from build123d import *

# Parameters (mm, degrees)
SKETCH1_W           = 119.38
SKETCH1_H           = 25.4
BOSS_EXTRUDE1_DEPTH = 46.355
SKETCH2_W           = 109.855
SKETCH2_H           = 83.185
CUT_EXTRUDE1_DEPTH  = 20.6375
FILLET1_R           = 2.54
FILLET2_R           = 2.54
SKETCH8_R           = 2.286
CUT_EXTRUDE2_DEPTH  = 20.32
SKETCH16_R          = 2.286
CUT_EXTRUDE4_DEPTH  = 20.32
SKETCH17_R          = 2.286
CUT_EXTRUDE5_DEPTH  = 20.32
SKETCH18_R          = 2.286
CUT_EXTRUDE6_DEPTH  = 20.32
SKETCH9_R           = 3.556
SKETCH9_R_2         = 2.286
BOSS_EXTRUDE2_DEPTH = 22.86
SKETCH11_R          = 3.556
SKETCH11_R_2        = 2.286
BOSS_EXTRUDE3_DEPTH = 22.86
SKETCH12_R          = 3.556
SKETCH12_R_2        = 2.286
BOSS_EXTRUDE4_DEPTH = 22.86
SKETCH13_R          = 3.556
SKETCH13_R_2        = 2.286
BOSS_EXTRUDE5_DEPTH = 22.86


with BuildPart() as part:
    # Sketch1 → Boss-Extrude1 (new body, symmetric)
    with BuildSketch(Plane.XY):
        with Locations((0, 12.7)):
            Rectangle(SKETCH1_W, SKETCH1_H)
    extrude(amount=BOSS_EXTRUDE1_DEPTH, both=True)

    # Sketch2 → Cut-Extrude1 (cut)
    with BuildSketch(Plane(origin=(0, 25.4, 0), x_dir=(1, 0, 0), z_dir=(0, 1, 0))):
        Rectangle(SKETCH2_W, SKETCH2_H)
    extrude(amount=-CUT_EXTRUDE1_DEPTH, mode=Mode.SUBTRACT)

    # Fillet1
    fillet1_edges = [part.edges().sort_by_distance(p)[0] for p in [
        (59.69, 12.7, 46.355),
        (-59.69, 12.7, 46.355),
        (59.69, 12.7, -46.355),
        (-59.69, 12.7, -46.355),
    ]]
    fillet(fillet1_edges, radius=FILLET1_R)

    # Fillet2
    fillet2_edges = [part.edges().sort_by_distance(p)[0] for p in [
        (59.69, 0, 0),
        (0, 0, -46.355),
        (0, 0, 46.355),
        (-59.69, 0, 0),
        (58.946051224, 0, 45.611051224),
        (-58.946051224, 0, 45.611051224),
        (-58.946051224, 0, -45.611051224),
        (58.946051224, 0, -45.611051224),
    ]]
    fillet(fillet2_edges, radius=FILLET2_R)

    # Sketch8 → Cut-Extrude2 (cut)
    with BuildSketch(Plane(origin=(0, 25.4, 0), x_dir=(1, 0, 0), z_dir=(0, 1, 0))):
        with Locations((56.896, 43.561)):
            Circle(SKETCH8_R)
    extrude(amount=-CUT_EXTRUDE2_DEPTH, mode=Mode.SUBTRACT)

    # Sketch16 → Cut-Extrude4 (cut)
    with BuildSketch(Plane(origin=(0, 25.4, 0), x_dir=(1, 0, 0), z_dir=(0, 1, 0))):
        with Locations((-56.896, -43.561)):
            Circle(SKETCH16_R)
    extrude(amount=-CUT_EXTRUDE4_DEPTH, mode=Mode.SUBTRACT)

    # Sketch17 → Cut-Extrude5 (cut)
    with BuildSketch(Plane(origin=(0, 25.4, 0), x_dir=(1, 0, 0), z_dir=(0, 1, 0))):
        with Locations((56.896, -43.561)):
            Circle(SKETCH17_R)
    extrude(amount=-CUT_EXTRUDE5_DEPTH, mode=Mode.SUBTRACT)

    # Sketch18 → Cut-Extrude6 (cut)
    with BuildSketch(Plane(origin=(0, 25.4, 0), x_dir=(1, 0, 0), z_dir=(0, 1, 0))):
        with Locations((-56.896, 43.561)):
            Circle(SKETCH18_R)
    extrude(amount=-CUT_EXTRUDE6_DEPTH, mode=Mode.SUBTRACT)

    # Sketch9 → Boss-Extrude2 (add)
    with BuildSketch(Plane(origin=(0, 4.7625, 0), x_dir=(1, 0, 0), z_dir=(0, 1, 0))):
        with Locations((-25.9715, 35.7505)):
            Circle(SKETCH9_R)
        with Locations((-25.9715, 35.7505)):
            Circle(SKETCH9_R_2, mode=Mode.SUBTRACT)
    extrude(amount=BOSS_EXTRUDE2_DEPTH)

    # Sketch11 → Boss-Extrude3 (add)
    with BuildSketch(Plane(origin=(0, 4.7625, 0), x_dir=(1, 0, 0), z_dir=(0, 1, 0))):
        with Locations((-30.8737, -32.8041)):
            Circle(SKETCH11_R)
        with Locations((-30.8737, -32.8041)):
            Circle(SKETCH11_R_2, mode=Mode.SUBTRACT)
    extrude(amount=BOSS_EXTRUDE3_DEPTH)

    # Sketch12 → Boss-Extrude4 (add)
    with BuildSketch(Plane(origin=(0, 4.7625, 0), x_dir=(1, 0, 0), z_dir=(0, 1, 0))):
        with Locations((47.8155, 35.8775)):
            Circle(SKETCH12_R)
        with Locations((47.8155, 35.8775)):
            Circle(SKETCH12_R_2, mode=Mode.SUBTRACT)
    extrude(amount=BOSS_EXTRUDE4_DEPTH)

    # Sketch13 → Boss-Extrude5 (add)
    with BuildSketch(Plane(origin=(0, 4.7625, 0), x_dir=(1, 0, 0), z_dir=(0, 1, 0))):
        with Locations((48.9585, -34.7345)):
            Circle(SKETCH13_R)
        with Locations((48.9585, -34.7345)):
            Circle(SKETCH13_R_2, mode=Mode.SUBTRACT)
    extrude(amount=BOSS_EXTRUDE5_DEPTH)


solid = part.part
Geometry check sheet. Reference: the model listing, model coordinates, mm. A direction names the side the tool comes from. Coordinates: 2 decimals unless noted, no trailing zeros. Order: outer loops, then holes, each group sorted by start corner. A loop starts at its lowest first (then second) coordinate and runs counter-clockwise, first axis right, second up. Notation, with made-up numbers: (7, -10.75) -> (19, -10.75) arc R16 ccw to (19, 19.25) -> close; hole circle Ø4 at (72.5, 68). An arc over 180 degrees is marked (long way). Use a Markdown table: item, result. Add a question column.
1. Set-up check for faces 4 (the face through (-59.69, 14, 1)), 5 (the face through (-1, 15, -41.592)): record each of +Z, -Z, +X, -X, +Y, -Y from which the full face is reachable in a straight line by a thin tool's end or side.
2. Cross-section at B-B (y = 22). Give the number of separate pieces and of enclosed holes in the cut face, and give its area (3 significant figures).
3. Material ranges on L1, parallel to Z at x = -18.5, y = 12.5 (1 decimal); L2, parallel to X at y = 11, z = -24.5; L3, parallel to Y at x = -11, z = -26.5, recorded low to high.
4. Go/stop test with flat-tipped pins: pin 1 Ø2.5 at (x, z) = (57, 43) entering from +Y; pin 2 Ø2.5 at (x, z) = (48.5, -35.5) entering from +Y; pin 3 Ø5.5 at (x, z) = (56.896, -43.561) entering from +Y. Record where each tip stops, or that it passes through.
5. Cross-section at A-A (z = 0). Enter the section's corners in (x, y).
6. Mould release check, pull along Z, two halves, no side actions. Record for faces 1 (the face through (59.69, 14, 1)), 2 (the face through (-57, 5.08, -44)), 3 (the face through (0.8, 0.724, -45.591)): pulls with the +Z half, pulls with the -Z half, needs draft (parallel to the pull), parting line crosses it, or undercut.
7. Cross-section at C-C (x = 16). Enter the section's corners in (y, z) (1 decimal).
Filled sheet:
| question | item | result |
|---|---|---|
| 1 | face 4 | +Z, -Z, -X, +Y, -Y |
| 1 | face 5 | +Y |
| 2 | separate pieces | 5 |
| 2 | enclosed holes | 9 |
| 2 | area | 1,950 mm2 |
| 3 | L1 | -46.4 to -41.6, 41.6 to 46.4 |
| 3 | L2 | -59.69 to -54.93, 54.93 to 59.69 |
| 3 | L3 | 0 to 4.76 |
| 4 | pin 1 | y = 5.08 |
| 4 | pin 2 | y = 4.76 |
| 4 | pin 3 | y = 25.4 |
| 5 | outline | (-59.69, 2.54) arc R2.54 ccw to (-57.15, 0) -> (57.15, 0) arc R2.54 ccw to (59.69, 2.54) -> (59.69, 25.4) -> (54.93, 25.4) -> (54.93, 4.76) -> (-54.93, 4.76) -> (-54.93, 25.4) -> (-59.69, 25.4) -> close |
| 6 | face 1 | needs draft |
| 6 | face 2 | undercut |
| 6 | face 3 | pulls with the -Z half |
| 7 | outline | (0, -43.8) arc R2.5 ccw to (2.5, -46.4) -> (25.4, -46.4) -> (25.4, -41.6) -> (4.8, -41.6) -> (4.8, 41.6) -> (25.4, 41.6) -> (25.4, 46.4) -> (2.5, 46.4) arc R2.5 ccw to (0, 43.8) -> close |
